Source: CAD feature listing. Evaluate the final solid. Frame: model axes, mm. A direction names the side the tool comes from. Give positions to 0.01 mm unless a question says otherwise; leave off trailing zeros. Order: outer loops, then holes, each group sorted by start corner. A loop starts at its lowest first (then second) coordinate and runs counter-clockwise, first axis right, second up. Notation, with made-up numbers: (44.25, 81.25) -> (80.25, 81.25) arc R13 ccw to (80.25, 106.25) -> close; hole circle Ø10 at (-17.75, -39). An arc over 180 degrees is marked (long way). Answer in a Markdown table with one row per item.
```python
from build123d import *

# Parameters (mm, degrees)
SKETCH2_W                    = 255.76
SKETCH2_H                    = 54.86
SKETCH2_W_2                  = 232.9
SKETCH2_H_2                  = 27.94
BASE_FLANGE1_DEPTH           = 1.27
EDGE_FLANGE1_STRIP_W         = 6.5532
EDGE_FLANGE1_STRIP_H         = 1.27
EDGE_FLANGE1_STRIP_CUT_DEPTH = 255.76
EDGE_FLANGE1_DEPTH           = 255.76
F_34_0_111_DIAMETER_HOLE1_D  = 2.8194
FILLET1_R                    = 2


# Sheet-metal steps are written as plain solids
with BuildPart() as part:
    # Sketch2 → Base-Flange1 (new body)
    with BuildSketch(Plane.XY):
        Rectangle(SKETCH2_W, SKETCH2_H)
        with Locations((0, 4.32)):
            Rectangle(SKETCH2_W_2, SKETCH2_H_2, mode=Mode.SUBTRACT)
    extrude(amount=-BASE_FLANGE1_DEPTH)

    # Edge-Flange1 strip (across the edge) → Edge-Flange1 strip cut (cut)
    with BuildSketch(Plane(origin=(127.88, -27.43, -1.27), x_dir=(0, 1, 0), z_dir=(-1, 0, 0))):
        with Locations((-1.27, -0.635)):
            Rectangle(EDGE_FLANGE1_STRIP_W, EDGE_FLANGE1_STRIP_H)
    extrude(amount=EDGE_FLANGE1_STRIP_CUT_DEPTH, mode=Mode.SUBTRACT)

    # Edge-Flange1 section (across the edge) → Edge-Flange1 (add)
    with BuildSketch(Plane(origin=(127.88, -27.43, -1.27), x_dir=(0, 1, 0), z_dir=(-1, 0, 0))):
        with BuildLine():
            Line((0, 0.7366), (0, 16.51))
            Line((0, 16.51), (1.27, 16.51))
            Line((1.27, 16.51), (1.27, 0.7366))
            ThreePointArc((1.27, 0.7366), (1.485745145, 0.215745145), (2.0066, 0))
            Line((2.0066, 0), (2.0066, -1.27))
            ThreePointArc((2.0066, -1.27), (0.587719533, -0.682280467), (0, 0.7366))
        make_face()
    extrude(amount=EDGE_FLANGE1_DEPTH)

    # #34 (0.111) Diameter Hole1 (through all)
    with Locations(Plane(origin=(0, 0, -1.27), x_dir=(-1, 0, 0), z_dir=(0, 0, -1))):
        with Locations((-122.95, 9.24), (121.16, 9.24)):
            Hole(F_34_0_111_DIAMETER_HOLE1_D / 2)

    # Fillet1
    fillet1_edges = [part.edges().sort_by_distance(p)[0] for p in [
        (127.88, -26.795, -17.78),
        (-127.88, -26.795, -17.78),
        (-127.88, 27.43, -0.635),
        (127.88, 27.43, -0.635),
    ]]
    fillet(fillet1_edges, radius=FILLET1_R)


solid = part.part
```
(1) Ray query, probe 1 along Y at (x, z) = (38.5, -16.5); probe 2 along Y at (x, z) = (-121.16, -0.65); probe 3 along Z at (x, y) = (77, -12). Return the intervals inside material, ascending.
A:
| item | result |
|---|---|
| probe 1 | y = -27.43 to -26.16 |
| probe 2 | y = -26.9 to 7.83, 10.65 to 27.43 |
| probe 3 | z = -1.27 to 0 |
(2) Section query C-C (y = -18). Return the cut outline in (x, z), plus the area to 3 significant figures.
A:
| item | result |
|---|---|
| outline | (-127.88, -1.27) -> (127.88, -1.27) -> (127.88, 0) -> (-127.88, 0) -> close |
| area | 325 mm^2 |
(3) First-contact query: pin 1 Ø5 at (x, z) = (20.5, -9) entering from +Y; pin 2 Ø3 at (x, y) = (-121.16, 9.24) entering from -Z. Flat tips, straight axial feed; report the tip coordinate or a pass-through.
A:
| item | result |
|---|---|
| pin 1 | stops at y = -26.16 |
| pin 2 | stops at z = -1.27 |
(4) Section query B-B (y = 16). Return the cut outline in (x, z), plus the area to 3 significant figures.
A:
| item | result |
|---|---|
| outline | (-127.88, -1.27) -> (-116.45, -1.27) -> (-116.45, 0) -> (-127.88, 0) -> close; (116.45, -1.27) -> (127.88, -1.27) -> (127.88, 0) -> (116.45, 0) -> close |
| area | 29.0 mm^2 |
(5) Section query A-A (x = 96). Return the cut outline in (y, z).
A:
| item | result |
|---|---|
| outline | (-27.43, -17.78) -> (-26.16, -17.78) -> (-26.16, -2.01) arc R0.74 cw to (-25.42, -1.27) -> (-9.65, -1.27) -> (-9.65, 0) -> (-25.42, 0) arc R2.01 ccw to (-27.43, -2.01) -> close; (18.29, -1.27) -> (27.43, -1.27) -> (27.43, 0) -> (18.29, 0) -> close |
(6) Access query for faces 1 (the flat face through (-2, -10, 0)), 2 (the flat face through (-2, -10, -1.27)). Directions: +Z, -Z, +X, -X, +Y, -Y. A direction counts if a zero-diameter tool reaches every point of the face in a straight line with its end or side. Return the directions, or none.
A:
| item | result |
|---|---|
| face 1 | +Z, +X, -X, +Y, -Y |
| face 2 | -Z, +X, -X, +Y |
(7) Section query D-D (z = -8.75). Return the cut outline in (x, y), plus the area to 3 significant figures.
A:
| item | result |
|---|---|
| outline | (-127.88, -27.43) -> (127.88, -27.43) -> (127.88, -26.16) -> (-127.88, -26.16) -> close |
| area | 325 mm^2 |
